Geometry: final body of the model. Coordinates: model frame, mm. A direction names the side the tool comes from. Coordinates: 2 decimals unless noted, no trailing zeros. Order: outer loops, then holes, each group sorted by start corner. A loop starts at its lowest first (then second) coordinate and runs counter-clockwise, first axis right, second up. Notation, with made-up numbers: (87, 35.5) -> (142, 35.5) arc R20 ccw to (142, 66.5) -> close; hole circle Ø2 at (45.25, -25). An arc over 180 degrees is marked (long way). Answer in a Markdown table with one row per item. Add a question column.
1) Set-up query: faces 4 (the face through (10.524, -12.003, 4.246)), 5 (the face through (10.68, -26, 10)), 6 (the face through (6, 0, 8.89)), 7 (the face through (11.43, 0, 7)). Return all of +Z, -Z, +X, -X, +Y, -Y with unobstructed straight access to the full face (end or side cutting, diameter ignored); none if empty.
2) Ray query, line 1 (Y direction, x = 0, z = 15); line 2 (Y direction, x = 3, z = 2.5); line 3 (Z direction, x = 0, y = -0.65). Return the intervals inside material, ascending. Write a range as from..to.
3) Pull-direction query (Y, two-part tool) for faces 1 (the face through (6, 7.62, 4)), 2 (the face through (10.107, -0.107, 1.255)), 3 (the face through (4, -17.76, 3.45)); classes: +Y half, -Y half, draft (parallel to the pull), parting line (faces both ways), or undercut.
4) Contact query for flat-ended pins moving along their axis: P1, Ø6, axis at x = 12, z = 11.5, coming from the -Y side; P2, Ø3, axis at x = 2.5, y = 3.5, coming from the -Z side; P3, Ø6, axis at x = -0.5, y = 0, coming from the +Z side; P4, Ø3, axis at y = -28.5, z = 10, coming from the +X side. Output: stop coordinate, or through.
5) Section query A-A on z = 28. Return the cut outline in (x, y).
```python
from build123d import *

# Parameters (mm, degrees)
MOVE_START             = 1.86
MOVE_FACE1_DEPTH       = 5.08
MOVE_FACE1_2_OUTLINE_R = 5.08
MOVE_FACE1_2_DEPTH     = 19.05
MOVE_FACE1_3_OUTLINE_R = 5.08
MOVE_FACE1_3_DEPTH     = 8.89
MOVE_START_2           = 19.05
MOVE_FACE1_4_OUTLINE_R = 2.95
MOVE_FACE1_4_DEPTH     = 19.05
MOVE_START_3           = 6.731
MOVE_FACE1_5_OUTLINE_R = 1.125
MOVE_FACE1_5_DEPTH     = 2.159
MOVE_START_4           = -7.62
MOVE_FACE1_6_OUTLINE_R = 1.27
MOVE_FACE1_6_DEPTH     = 15.24
MOVE_START_5           = -19.05
MOVE_FACE1_7_OUTLINE_R = 3.81
MOVE_FACE1_7_DEPTH     = 11.43
CUT_EXTRUDE2_START     = -8.3
SKETCH4_R              = 3.75
SKETCH4_R_2            = 2.95
CUT_EXTRUDE2_DEPTH     = 8.3
MOVE_FACE2_BY          = 0.08
SKETCH6_W              = 22.532040778
SKETCH6_H              = 17.162622236
CUT_EXTRUDE3_DEPTH     = 16.1
SKETCH7_W              = 16.875
SKETCH7_H              = 7.3
BOSS_EXTRUDE1_DEPTH    = 14.2
CUT_EXTRUDE4_DEPTH     = 14.2
MOVE_START_6           = 3.38
MOVE_FACE5_DEPTH       = 7.3
CUT_EXTRUDE5_REACH     = 50.258


with BuildPart() as part:
    # Move Face1: read off the stored shape, not the designer's step
    # Move Face1 outline → Move Face1 (new body)
    with BuildSketch(Plane.XY.offset(MOVE_START)):
        with BuildLine():
            ThreePointArc((-3.511, -31.99383827), (7.03, -34.29), (17.571, -31.99383827))
            Line((17.571, -31.99383827), (17.571, -22.753852444))
            Line((17.571, -22.753852444), (11.389315764, -19.05))
            Line((11.389315764, -19.05), (2.670684236, -19.05))
            Line((2.670684236, -19.05), (-3.511, -22.753852444))
            Line((-3.511, -22.753852444), (-3.511, -31.99383827))
        make_face()
        with BuildLine():
            Line((0, -7.62), (11.43, -7.62))
            Line((11.43, -7.62), (11.43, 7.62))
            Line((11.43, 7.62), (0, 7.62))
            ThreePointArc((0, 7.62), (-7.62, 0), (0, -7.62))
        make_face()
    extrude(amount=MOVE_FACE1_DEPTH)

    # Move Face1 2 outline → Move Face1 2 (add)
    with BuildSketch(Plane.XY):
        Circle(MOVE_FACE1_2_OUTLINE_R)
    extrude(amount=MOVE_FACE1_2_DEPTH)

    # Move Face1 3 outline → Move Face1 3 (add)
    with BuildSketch(Plane.XY):
        with BuildLine():
            ThreePointArc((0, 7.62), (-7.62, 0), (0, -7.62))
            Line((0, -7.62), (11.43, -7.62))
            Line((11.43, -7.62), (11.43, 7.62))
            Line((11.43, 7.62), (0, 7.62))
        make_face()
        Circle(MOVE_FACE1_3_OUTLINE_R, mode=Mode.SUBTRACT)
    extrude(amount=MOVE_FACE1_3_DEPTH)

    # Move Face1 4 outline → Move Face1 4 (add)
    with BuildSketch(Plane.XY.offset(MOVE_START_2)):
        Circle(MOVE_FACE1_4_OUTLINE_R)
    extrude(amount=MOVE_FACE1_4_DEPTH)

    # Move Face1 5 outline → Move Face1 5 (add)
    with BuildSketch(Plane.XY.offset(MOVE_START_3)):
        with BuildLine():
            Line((-10.24004056, 5.820733333), (-7.414650266, 1.75708891))
            ThreePointArc((-7.414650266, 1.75708891), (-5.388153673, 5.388153673), (-1.75708891, 7.414650266))
            Line((-1.75708891, 7.414650266), (-5.820733333, 10.24004056))
            ThreePointArc((-5.820733333, 10.24004056), (-9.878281733, 9.878281733), (-10.24004056, 5.820733333))
        make_face()
        with Locations((-7.633217703, 7.633217703)):
            Circle(MOVE_FACE1_5_OUTLINE_R, mode=Mode.SUBTRACT)
    extrude(amount=MOVE_FACE1_5_DEPTH)

    # Move Face1 6 outline → Move Face1 6 (cut)
    with BuildSketch(Plane(origin=(0, 0, 0), x_dir=(1, 0, 0), z_dir=(0, 1, 0)).offset(MOVE_START_4)):
        with BuildLine():
            ThreePointArc((7.03, 0), (10.141269837, -1.288730163), (11.43, -4.4))
            Line((11.43, -4.4), (11.43, 0))
            Line((11.43, 0), (7.03, 0))
        make_face()
        with Locations((0, -32.4485)):
            Circle(MOVE_FACE1_6_OUTLINE_R)
    extrude(amount=MOVE_FACE1_6_DEPTH, mode=Mode.SUBTRACT)

    # Move Face1 7 outline → Move Face1 7 (add)
    with BuildSketch(Plane(origin=(0, 0, 0), x_dir=(1, 0, 0), z_dir=(0, 1, 0)).offset(MOVE_START_5)):
        with Locations((7.03, -4.4)):
            Circle(MOVE_FACE1_7_OUTLINE_R)
    extrude(amount=MOVE_FACE1_7_DEPTH)

    # Move Face1 8 outline → Move Face1 8 (revolve, cut)
    with BuildSketch(Plane.XZ):
        with BuildLine():
            ThreePointArc((0, 38.1), (1.499969695, 37.962580669), (2.95, 37.554897859))
            Line((2.95, 37.554897859), (2.95, 38.1))
            Line((2.95, 38.1), (0, 38.1))
        make_face()
        with BuildLine():
            Line((2.95, 27.392283801), (2.95, 37.504716198))
            ThreePointArc((2.95, 37.504716198), (2.061, 32.448499999), (2.95, 27.392283801))
        make_face()
    revolve(axis=Axis((0, 0, 0), (0, 0, 1)), mode=Mode.SUBTRACT)

    # Move Face1 9 outline → Move Face1 9 (revolve)
    with BuildSketch(Plane.XZ):
        with BuildLine():
            ThreePointArc((2.95, 37.504716198), (2.958008721, 37.526732793), (2.96605223, 37.548736702))
            ThreePointArc((2.96605223, 37.548736702), (2.958027723, 37.551821458), (2.95, 37.554897859))
            Line((2.95, 37.554897859), (2.95, 37.504716198))
        make_face()
    revolve(axis=Axis((0, 0, 0), (0, 0, 1)))

    # Sketch4 → Cut-Extrude2 (cut)
    with BuildSketch(Plane.XY.offset(19.05).offset(CUT_EXTRUDE2_START)):
        Circle(SKETCH4_R)
        Circle(SKETCH4_R_2, mode=Mode.SUBTRACT)
    extrude(amount=CUT_EXTRUDE2_DEPTH, mode=Mode.SUBTRACT)

    # Sketch5 → Cut-Revolve1 (revolve, cut)
    with BuildSketch(Plane(origin=(0, 0, 4.4), x_dir=(-1, 0, 0), z_dir=(0, 0, -1))):
        Polygon((-3.22, -7.62), (-3.22, -19.05), (-3.855, -19.05), (-3.855, -16.51), align=None)
    revolve(axis=Axis((7.03, -7.62, 4.4), (0, -1, 0)), mode=Mode.SUBTRACT)

    # Move Face2: a curved face moved inward by 0.08
    add(Solid.thicken(part.faces().sort_by_distance((-5.08, 0, 13.97))[0], -MOVE_FACE2_BY), mode=Mode.SUBTRACT)

    # Sketch6 → Cut-Extrude3 (cut)
    with BuildSketch(Plane.XY):
        with Locations((7.03, -27.631311118)):
            Rectangle(SKETCH6_W, SKETCH6_H)
    extrude(amount=CUT_EXTRUDE3_DEPTH, mode=Mode.SUBTRACT)

    # Sketch7 → Boss-Extrude1 (add)
    with BuildSketch(Plane.XZ.offset(19.05)):
        with Locations((7.03, 4.4)):
            Rectangle(SKETCH7_W, SKETCH7_H)
    extrude(amount=BOSS_EXTRUDE1_DEPTH)

    # Sketch8 → Cut-Extrude4 (cut)
    with BuildSketch(Plane(origin=(0, 0, 0.75), x_dir=(-1, 0, 0), z_dir=(0, 0, -1))):
        with BuildLine():
            Line((-10.205, -19.571854416), (-10.205, -19.05))
            Line((-10.205, -19.05), (-15.4675, -19.05))
            Line((-15.4675, -19.05), (-15.4675, -26.15))
            add(Edge.make_bspline(
                [(-10.205, -19.571854416), (-15.4675, -21.370400141), (-15.4675, -26.15)],
                knots=[1.956591838, 1.956591838, 1.956591838, 3.141592654, 3.141592654, 3.141592654], degree=2, weights=[1, 0.829546954, 1]))
        make_face()
        with BuildLine():
            Line((1.4075, -19.05), (-3.855, -19.05))
            Line((-3.855, -19.05), (-3.855, -19.571854416))
            add(Edge.make_bspline(
                [(1.4075, -26.15), (1.4075, -21.370400141), (-3.855, -19.571854416)],
                knots=[0, 0, 0, 1.185000816, 1.185000816, 1.185000816], degree=2, weights=[1, 0.829546954, 1]))
            Line((1.4075, -26.15), (1.4075, -19.05))
        make_face()
        with BuildLine():
            add(Edge.make_bspline(
                [(-15.4675, -26.15), (-15.4675, -33.25), (-7.03, -33.25)],
                knots=[3.141592654, 3.141592654, 3.141592654, 4.71238898, 4.71238898, 4.71238898], degree=2, weights=[1, 0.707106781, 1]))
            Line((-15.4675, -26.15), (-15.4675, -33.25))
            Line((-15.4675, -33.25), (-7.03, -33.25))
        make_face()
        with BuildLine():
            Line((1.4075, -33.25), (1.4075, -26.15))
            add(Edge.make_bspline(
                [(-7.03, -33.25), (1.4075, -33.25), (1.4075, -26.15)],
                knots=[4.71238898, 4.71238898, 4.71238898, 6.283185307, 6.283185307, 6.283185307], degree=2, weights=[1, 0.707106781, 1]))
            Line((-7.03, -33.25), (1.4075, -33.25))
        make_face()
    extrude(amount=-CUT_EXTRUDE4_DEPTH, mode=Mode.SUBTRACT)

    # Move Face5: read off the stored shape, not the designer's step
    # Move Face5 outline → Move Face5 (add)
    with BuildSketch(Plane.YZ.offset(MOVE_START_6)):
        with BuildLine():
            Line((-32.551285538, 0.75), (-19.748714462, 0.75))
            add(Edge.make_bspline(
                [(-19.748714462, 0.75), (-19.654129969, 0.984263783), (-19.571854416, 1.225)],
                knots=[1.123429947, 1.123429947, 1.123429947, 1.185000816, 1.185000816, 1.185000816], degree=2, weights=[1, 0.999526166, 1]))
            Line((-19.571854416, 1.225), (-19.05, 1.225))
            Line((-19.05, 1.225), (-19.05, 7.575))
            Line((-19.05, 7.575), (-19.571854416, 7.575))
            add(Edge.make_bspline(
                [(-19.571854416, 7.575), (-19.654129969, 7.815736217), (-19.748714462, 8.05)],
                knots=[1.956591838, 1.956591838, 1.956591838, 2.018162706, 2.018162706, 2.018162706], degree=2, weights=[1, 0.999526166, 1]))
            Line((-19.748714462, 8.05), (-32.551285538, 8.05))
            add(Edge.make_bspline(
                [(-32.551285538, 8.05), (-34.02498069, 4.4), (-32.551285538, 0.75)],
                knots=[4.265022601, 4.265022601, 4.265022601, 5.15975536, 5.15975536, 5.15975536], degree=2, weights=[1, 0.901589512, 1]))
        make_face()
        with BuildLine():
            add(Edge.make_bspline(
                [(-32.551285538, 0.75), (-26.15, -15.104494863), (-19.748714462, 0.75)],
                knots=[5.15975536, 5.15975536, 5.15975536, 7.406615254, 7.406615254, 7.406615254], degree=2, weights=[1, 0.432592593, 1]))
            Line((-19.748714462, 0.75), (-32.551285538, 0.75))
        make_face()
        with BuildLine():
            add(Edge.make_bspline(
                [(-19.748714462, 8.05), (-26.15, 23.904494863), (-32.551285538, 8.05)],
                knots=[2.018162706, 2.018162706, 2.018162706, 4.265022601, 4.265022601, 4.265022601], degree=2, weights=[1, 0.432592593, 1]))
            Line((-32.551285538, 8.05), (-19.748714462, 8.05))
        make_face()
    extrude(amount=MOVE_FACE5_DEPTH)

    # Sketch10 → Cut-Extrude5 (cut, up to next)
    with BuildSketch(Plane(origin=(0, 0, 6.731), x_dir=(-1, 0, 0), z_dir=(0, 0, -1)), mode=Mode.PRIVATE) as cut_extrude5_sk1:
        with BuildLine():
            Line((5.820733333, 10.24004056), (1.75708891, 7.414650266))
            ThreePointArc((1.75708891, 7.414650266), (5.388153673, 5.388153673), (7.414650266, 1.75708891))
            Line((7.414650266, 1.75708891), (10.24004056, 5.820733333))
            ThreePointArc((10.24004056, 5.820733333), (9.878281733, 9.878281733), (5.820733333, 10.24004056))
        make_face()
    cut_extrude5_tool1 = extrude(cut_extrude5_sk1.sketch, amount=-CUT_EXTRUDE5_REACH, mode=Mode.PRIVATE) & part.part
    add(cut_extrude5_tool1.solids().sort_by_distance((-7.209511, 7.209511, 6.731))[0], mode=Mode.SUBTRACT)


solid = part.part
```
Result:
| question | item | result |
|---|---|---|
| 1 | face 4 | none |
| 1 | face 5 | +Z, +X, -Y |
| 1 | face 6 | +Z |
| 1 | face 7 | +Z, -Z, +X, +Y |
| 2 | line 1 | -5..-3.75, -2.95..2.95, 3.75..5 |
| 2 | line 2 | -32.39..-19.91, -7.62..7.62 |
| 2 | line 3 | 0..31.18, 33.72..38.07 |
| 3 | face 1 | +Y half |
| 3 | face 2 | draft |
| 3 | face 3 | undercut |
| 4 | P1 | y = -32.21 |
| 4 | P2 | z = 0 |
| 4 | P3 | z = 38.1 |
| 4 | P4 | x = 10.68 |
| 5 | outline | circle Ø5.49 at (0, 0) |
